Autodesk Inventor part; units mm, degrees
ref_plane "YZ Plane" through (0, 0, 0) normal (1, 0, 0) x (0, 1, 0)
ref_plane "XZ Plane" through (0, 0, 0) normal (0, 1, 0) x (-1, 0, 0)
ref_plane "XY Plane" through (0, 0, 0) normal (0, 0, 1) x (1, 0, 0)
sketch "Sketch1" plane through (0, 0, 0) normal (0, 1, 0) x (-1, 0, 0)
  line L0 (50, 80) -> (-50, 80) construction
  line L1 (-50, 80) -> (-50, -80) construction
  line L2 (-50, -80) -> (50, -80) construction
  line L3 (50, -80) -> (50, 80) construction
  line L4 (50, -80) -> (40, -80)
  line L5 (40, -80) -> (40, -50)
  line L6 (50, -80) -> (50, -50)
  line L7 (-50, 80) -> (-50, 60)
  line L8 (-50, 80) -> (-40, 80)
  line L9 (-40, 80) -> (-40, 60)
  line L10 (-40, 60) -> (50, -50)
  line L11 (-50, 60) -> (40, -50)
  point P0 (0, 0)
  point P1 (50, 0)
  point P2 (0, -80)
  dimension "d0" = 160
  dimension "d1" = 100
  dimension "d2" = 10
  dimension "d3" = 30
  dimension "d4" = 20
  dimension "d5" = 10
extrude "Extrusion1" add sketch "Sketch1" along normal blind 10
sketch "Sketch2" plane through (40, 0, 80) normal (0, 0, 1) x (1, 0, 0)
  line L0 (-90, 0) -> (0, 0) construction
  line L1 (10, 10) -> (-80, 10) construction
  line L2 (0, 0) -> (10, 10) construction
  line L3 (2.5, 7.5) -> (7.5, 7.5)
  line L4 (7.5, 7.5) -> (7.5, 2.5)
  line L5 (7.5, 2.5) -> (2.5, 2.5)
  line L6 (2.5, 2.5) -> (2.5, 7.5)
  line L7 (2.5, 7.5) -> (7.5, 2.5) construction
  line L8 (7.5, 7.5) -> (2.5, 2.5) construction
  point P0 (-40, 0)
  point P1 (5, 5)
  dimension "d8" = 5
  dimension "d9" = 5
extrude "Extrusion2" cut sketch "Sketch2" against normal blind 15
sketch "Sketch4" plane through (0, 10, 0) normal (0, 1, 0) x (1, 0, 0)
  line L0 (50, -80) -> (50, -60)
  line L1 (50, -60) -> (-84.9338, -60)
  line L2 (-84.9338, -60) -> (-84.9338, 89.9806)
  line L3 (-84.9338, 89.9806) -> (50, 89.9806)
  line L4 (50, 89.9806) -> (50, -60)
  point P0 (0, 0)
extrude "Extrusion4" cut sketch "Sketch4" against normal blind 10
sketch "Sketch5" plane through (50, 10, 60) normal (0, 0, -1) x (-1, 0, 0)
  line L0 (0, -10) -> (0, 0)
  line L1 (10, -10) -> (10, 0)
  line L2 (0, -10) -> (10, -10)
  line L3 (10, -10) -> (10, 0)
  line L4 (10, 0) -> (0, 0)
  line L5 (0, 0) -> (0, -10)
  point P0 (50, -10)
extrude "Extrusion5" add sketch "Sketch5" along normal blind 10
sketch "Sketch7" plane through (50, 10, 50) normal (0, 0, -1) x (-1, 0, 0)
  line L0 (0, 0) -> (0, -10)
  line L1 (10, 0) -> (0, 0)
  line L2 (0, -10) -> (10, -10)
  line L3 (10, -10) -> (10, 0)
  line L4 (10, 0) -> (0, 0)
  line L5 (0, 0) -> (0, -10)
  point P0 (50, -10)
extrude "Extrusion6" add sketch "Sketch7" along normal blind 27
sketch "Sketch9" plane through (0, 10, 0) normal (0, 1, 0) x (1, 0, 0)
  arc A0 (46.9, -28) -> (43.1, -28) centre (45, -28) ccw
  line L0 (40, -23) -> (50, -23)
  arc A1 (43.1, -44) -> (46.9, -44) centre (45, -44) ccw
  line L1 (40, -80) -> (40, -23)
  line L2 (43.1, -44) -> (43.1, -28)
  line L3 (46.9, -44) -> (46.9, -28)
  point P0 (0, 0)
  dimension "d25" = 3.8
  dimension "d26" = 5
  dimension "d27" = 3.8
  dimension "d28" = 16
  dimension "d29" = 5
extrude "Extrusion7" cut sketch "Sketch9" against normal blind 5
properties part number "Arm_v2_richard"
Input: part model. Units: mm. Frame: model coordinates. A direction names the side the tool comes from. Coordinates: 2 decimals unless noted, no trailing zeros. Order: outer loops, then holes, each group sorted by start corner. A loop starts at its lowest first (then second) coordinate and runs counter-clockwise, first axis right, second up. Notation, with made-up numbers: M 64.25,-36.75 L 94.25,-36.75 A28 cw 94.25,-10.75 Z; hole C -37.5,51 d10. An arc over 180 degrees is marked long. One line per question, with ' | ' between items.
Item 1: Ray query, line 1 along X through (y, z) = (7, 36.5); line 2 along X through (y, z) = (2.75, 74); line 3 along Y through (x, z) = (46, 71.5). Return the intervals inside material, ascending.
Geometry results:
line 1: x = 40 to 43.1, 46.9 to 50 | line 2: x = 40 to 42.5, 47.5 to 50 | line 3: y = 0 to 2.5, 7.5 to 10
Item 2: Section A-A (y = 8.25). Output: boundary loops of the cut face in (x, z), then the cut area to 3 significant figures.
Geometry results:
outline: M 40,23 L 50,23 L 50,80 L 40,80 Z; hole M 43.1,28 A1.9 ccw 46.9,28 L 46.9,44 A1.9 ccw 43.1,44 Z | area: 498 mm^2
Item 3: Section D-D (x = 44.75). Output: boundary loops of the cut face in (y, z).
Geometry results:
outline: M 0,23 L 10,23 L 10,26.12 L 5,26.12 L 5,45.88 L 10,45.88 L 10,80 L 7.5,80 L 7.5,65 L 2.5,65 L 2.5,80 L 0,80 Z
Item 4: Section B-B (z = 74.5). Output: boundary loops of the cut face in (x, y), then the cut area to 3 significant figures.
Geometry results:
outline: M 40,0 L 50,0 L 50,10 L 40,10 Z; hole M 42.5,2.5 L 47.5,2.5 L 47.5,7.5 L 42.5,7.5 Z | area: 75.0 mm^2
Item 5: Section C-C (y = 4). Output: boundary loops of the cut face in (x, z).
Geometry results:
outline: M 40,23 L 50,23 L 50,80 L 47.5,80 L 47.5,65 L 42.5,65 L 42.5,80 L 40,80 Z
Item 6: Pin query (flat end, axial travel): pin 1 (1.5 mm diameter, centred on x = 44, y = 5, fed in from +Z); pin 2 (1.9 mm diameter, centred on x = 45.5, z = 35, fed in from +Y). Return the tip coordinate at first contact, or that it passes through.
Geometry results:
pin 1: stops at z = 65 | pin 2: stops at y = 5
Item 7: Reachability of faces 1 (the flat face through (45, 2.5, 73)), 2 (the cylindrical face through (45, 7.5, 45.9)), 3 (the flat face through (40, 5, 52)) from +Z, -Z, +X, -X, +Y, -Y: full face, straight path, thin tool, end or side. Return the list, or none.
Geometry results:
face 1: +Z | face 2: +Y | face 3: +Z, -Z, -X, +Y, -Y
Item 8: Draft query along X for faces 4 (the flat face through (50, 5, 52)), 5 (the flat face through (47.5, 5, 73)), 6 (the flat face through (42.5, 5, 73)), 7 (the flat face through (42, 5, 80)). Return one class per face: released by +X, released by -X, zero draft, split by the parting line, or undercut.
Geometry results:
face 4: released by +X | face 5: undercut | face 6: undercut | face 7: zero draft
